Design review of the part built by this model. Coordinates are the model's own, in mm. Face numbers are marked on the shaded views. A direction names the side the tool comes from. Coordinates: 2 decimals unless noted, no trailing zeros. Write each loop counter-clockwise with the first axis right and the second up, starting at its lowest first coordinate (ties: lowest second). Pieces come first, ordered by that corner, then holes.
Q1. Mouldability with a two-part tool opening along X and no side actions: class the marked faces 3, 4 and 5 as pulls with the +X half, pulls with the -X half, needs draft (parallel to the pull), parting line crosses it, or undercut.
Q2. Insertion check: pin 1 (5 mm diameter, centred on y = -279, z = 335, fed in from +X); pin 2 (5 mm diameter, centred on x = -532, y = -99.5, fed in from -Z). Each pin has a flat end and moves straight along its axis. Give the tip position at first contact, or say it passes through.
Q3. Machinability: for the marked faces 1 and 2, which of the approach directions +Z, -Z, +X, -X, +Y, -Y give a long, thin tool a straight path to every point of the face, cutting with its end or side? Answer none if there is none.
Q4. Take a section at C-C (y = 306.5). Give the boundary of the cut face in (x, z), and give its area (3 significant figures).
Q5. Take a section at A-A (y = -28). Give the boundary of the cut face in (x, z).
Q6. For probe 1 along X at (y, z) = (273, 798); probe 2 along Z at (x, y) = (-132, 43), list the stretches that pass through material, from the lowest coordinate up.
Q7. Take a section at B-B (z = 718). Give the boundary of the cut face in (x, y), and give its area (3 significant figures).
Q8. Take a section at D-D (x = -916). Give the boundary of the cut face in (y, z), and give its area (3 significant figures).
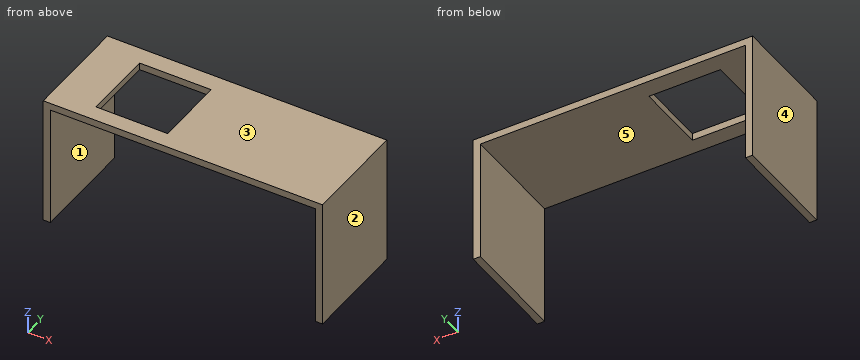
```python
from build123d import *

# Parameters (mm, degrees)
F0_W     = 1981.2
F0_H     = 914.4
F1_DEPTH = 374.65
F2_W     = 1879.6
F2_H     = 863.6
F3_DEPTH = 749.301
F4_W     = 508
F4_H     = 508
F5_DEPTH = 914.401


with BuildPart() as f1:
    # F0 (on Front) → F1 (new body, symmetric)
    with BuildSketch(Plane.XZ):
        with Locations((-990.6, 457.2)):
            Rectangle(F0_W, F0_H)
    extrude(amount=F1_DEPTH, both=True)

    # F2 (on face) → F3 (cut, through all)
    with BuildSketch(Plane.XZ.offset(374.65)):
        with Locations((-990.6, 431.8)):
            Rectangle(F2_W, F2_H)
    extrude(amount=-F3_DEPTH, mode=Mode.SUBTRACT)

    # F4 (on face) → F5 (cut, through all)
    with BuildSketch(Plane.XY.offset(914.4)):
        with Locations((-1422.4, -6.35)):
            Rectangle(F4_W, F4_H)
    extrude(amount=-F5_DEPTH, mode=Mode.SUBTRACT)


solid = f1.part
```
Response:
1. face 3: needs draft
1. face 4: pulls with the -X half
1. face 5: undercut
2. pin 1: stops at x = 0
2. pin 2: stops at z = 863.6
3. face 1: -Z, +Y, -Y
3. face 2: +Z, -Z, +X, +Y, -Y
4. outline: (-1981.2, 0) - (-1930.4, 0) - (-1930.4, 863.6) - (-50.8, 863.6) - (-50.8, 0) - (0, 0) - (0, 914.4) - (-1981.2, 914.4) - close
4. area: 188,000 mm2
5. outline: (-1981.2, 0) - (-1930.4, 0) - (-1930.4, 863.6) - (-1676.4, 863.6) - (-1676.4, 914.4) - (-1981.2, 914.4) - close; (-1168.4, 863.6) - (-50.8, 863.6) - (-50.8, 0) - (0, 0) - (0, 914.4) - (-1168.4, 914.4) - close
6. probe 1: x = -1981.2 to -1930.4, -50.8 to 0
6. probe 2: z = 863.6 to 914.4
7. outline: (-1981.2, -374.65) - (-1930.4, -374.65) - (-1930.4, 374.65) - (-1981.2, 374.65) - close; (-50.8, -374.65) - (0, -374.65) - (0, 374.65) - (-50.8, 374.65) - close
7. area: 76,100 mm2
8. outline: (-374.65, 863.6) - (374.65, 863.6) - (374.65, 914.4) - (-374.65, 914.4) - close
8. area: 38,100 mm2
